Design review of the part built by this model. Coordinates are the model's own, in mm. Coordinates: 2 decimals unless noted, no trailing zeros. Order: outer loops, then holes, each group sorted by start corner. A loop starts at its lowest first (then second) coordinate and runs counter-clockwise, first axis right, second up. Notation, with made-up numbers: (18.25, -18) -> (44.25, -18) arc R23 cw to (44.25, -9) -> close; hole circle Ø7 at (54.25, 12.25). An arc over 180 degrees is marked (long way). Use a Markdown table: item, result. Add a question column.
Q1. Wall thickness on probe 1 along X at (y, z) = (1.2, -2.5); probe 2 along X at (y, z) = (7.5, -2.5); probe 3 along Z at (x, y) = (-6.5, 7.25): over which ranges is each line inside the solid? List them lowest first.
Q2. The part is to be moulded in two halves that separate along Z. For faces 1 (the face through (-0.285, 5.1, -4.699)), 2 (the face through (-7, 5, 0)), 3 (the face through (-8.483, 6.481, -2.76)), say which applies: pulls with the +Z half, pulls with the -Z half, needs draft (parallel to the pull), parting line crosses it, or undercut.
Q3. Add section D-D (y = 5.5). State the section outline as (x, z) points, then the cut area to 3 significant figures.
Q4. Add section A-A (x = -6.5). State the section outline as (y, z) points, then the cut area to 3 significant figures.
Q5. Add section C-C (y = 2.75). State the section outline as (x, z) points, then the cut area to 3 significant figures.
Q6. Insertion check: pin 1 (1.4 mm diameter, centred on x = -6.5, z = -2.5, fed in from +Y); pin 2 (2 mm diameter, centred on x = -6, z = -3, fed in from +Y). Each pin has a flat end and moves straight along its axis. Give the tip position at first contact, or say it passes through.
Q7. Add section B-B (z = -2.5). State the section outline as (x, y) points, then the cut area to 3 significant figures.
Autodesk Inventor part; units mm, degrees
ref_plane "YZ Plane" through (0, 0, 0) normal (1, 0, 0) x (0, 1, 0)
ref_plane "XZ Plane" through (0, 0, 0) normal (0, 1, 0) x (-1, 0, 0)
ref_plane "XY Plane" through (0, 0, 0) normal (0, 0, 1) x (1, 0, 0)
sketch "Boceto1" plane through (0, 0, 0) normal (0, 1, 0) x (-1, 0, 0)
  line L0 (0, 0) -> (0, -5)
  line L1 (0, -5) -> (13, -5)
  line L2 (13, -5) -> (13, 0)
  line L3 (13, 0) -> (0, 0)
  circle A0 centre (6.5, -2.5) radius 0.9
  dimension "d0" = 5
  dimension "d1" = 13
  dimension "d2" = 1.8
extrude "Extrusión1" add sketch "Boceto1" along normal blind 10.06
sketch "Boceto2" plane through (0, 10.06, 0) normal (0, 1, 0) x (1, 0, 0)
  circle A0 centre (-6.5, 2.5) radius 0.9
  point P0 (0, 0)
hole "Agujero1" at (-6.5, 10.06, -2.5) direction (0, -1, 0) diameter 4 depth 7.06
fillet "Empalme1" radius 1 4 edges at (0, 5.03, 0) (0, 5.03, -5) (-13, 5.03, 0) (-13, 5.03, -5)
properties part number "Soporte placa 2.0"
Established:
| question | item | result |
|---|---|---|
| 1 | probe 1 | -13 to -7.4, -5.6 to 0 |
| 1 | probe 2 | -13 to -8.5, -4.5 to 0 |
| 1 | probe 3 | -5 to -4.5, -0.5 to 0 |
| 2 | face 1 | pulls with the -Z half |
| 2 | face 2 | pulls with the +Z half |
| 2 | face 3 | undercut |
| 3 | outline | (-13, -4) arc R1 ccw to (-12, -5) -> (-1, -5) arc R1 ccw to (0, -4) -> (0, -1) arc R1 ccw to (-1, 0) -> (-12, 0) arc R1 ccw to (-13, -1) -> close; hole circle Ø4 at (-6.5, -2.5) |
| 3 | area | 51.6 mm^2 |
| 4 | outline | (0, -5) -> (10.06, -5) -> (10.06, -4.5) -> (3, -4.5) -> (3, -3.4) -> (0, -3.4) -> close; (0, -1.6) -> (3, -1.6) -> (3, -0.5) -> (10.06, -0.5) -> (10.06, 0) -> (0, 0) -> close |
| 4 | area | 16.7 mm^2 |
| 5 | outline | (-13, -4) arc R1 ccw to (-12, -5) -> (-1, -5) arc R1 ccw to (0, -4) -> (0, -1) arc R1 ccw to (-1, 0) -> (-12, 0) arc R1 ccw to (-13, -1) -> close; hole circle Ø1.8 at (-6.5, -2.5) |
| 5 | area | 61.6 mm^2 |
| 6 | pin 1 | through |
| 6 | pin 2 | y = 3 |
| 7 | outline | (-13, 0) -> (-7.4, 0) -> (-7.4, 3) -> (-8.5, 3) -> (-8.5, 10.06) -> (-13, 10.06) -> close; (-5.6, 0) -> (0, 0) -> (0, 10.06) -> (-4.5, 10.06) -> (-4.5, 3) -> (-5.6, 3) -> close |
| 7 | area | 97.1 mm^2 |
